Here's how the part is built. I have some questions about the finished solid (model axes, mm). Face numbers are marked on the shaded views. A direction names the side the tool comes from. Round coordinates to 2 decimals unless told otherwise and drop trailing zeros. Write each loop counter-clockwise with the first axis right and the second up, starting at its lowest first coordinate (ties: lowest second). Pieces come first, ordered by that corner, then holes. Notation, with made-up numbers: (55, 77) - (110, 77) arc R14 cw to (110, 91) - close; hole circle Ø10 at (-33, 88). An arc over 180 degrees is marked (long way). One line per item, written item: value. Start each with the question number.
Item 1: For P1, Ø7, axis at x = 0, z = 0, coming from the -Y side; P2, Ø2, axis at y = -2, z = 3, coming from the +X side; P3, Ø1, axis at x = 5, z = 7.5, coming from the +Y side, each with a flat end and sliding along its axis, tell me the tip position at first contact or that it passes through.
Item 2: Imagine slicing it at C-C, the plane y = 2.75. Please give me the cut outline in (x, z), then the cut area to 3 significant figures.
Item 3: If I drill on line 1 (X direction, y = -3.75, z = 0); line 2 (X direction, y = 2.5, z = 0); line 3 (Z direction, x = -7, y = 3.5), over which ranges is the centre line in solid material (lowest first)?
Item 4: Thinking about a two-plate mould opening in Z: for the marked faces 1, 2 and 3, which applies, released by +Z, released by -Z, zero draft, split by the parting line, or undercut?
Item 5: For the marked faces 4 and 5, which set-ups out of +Z, -Z, +X, -X, +Y, -Y let a thin tool reach every point of the face, with its end or its side?
Item 6: Imagine slicing it at D-D, the plane x = 4.75. Please give me the cut outline in (y, z).
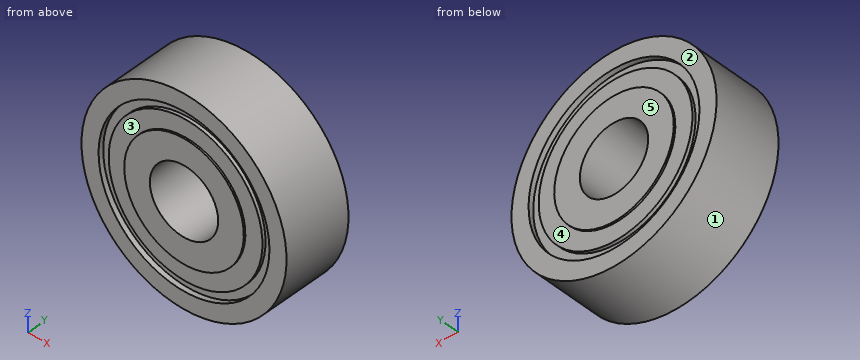
```python
from build123d import *

# Parameters (mm, degrees)
SKETCH1_R           = 7
SKETCH1_R_2         = 4
BOSS_EXTRUDE1_DEPTH = 4
SKETCH3_R           = 9
SKETCH3_R_2         = 7
BOSS_EXTRUDE2_DEPTH = 3.8
SKETCH4_R           = 10
SKETCH4_R_2         = 9
BOSS_EXTRUDE3_DEPTH = 3.4
SKETCH5_R           = 12
SKETCH5_R_2         = 10
BOSS_EXTRUDE4_DEPTH = 4


with BuildPart() as part:
    # Sketch1 → Boss-Extrude1 (new, symmetric)
    with BuildSketch(Plane(origin=(0, 0, 0), x_dir=(1, 0, 0), z_dir=(0, 1, 0))):
        with Locations(Location((0, 0, 0), (0, 0, 270))):
            Circle(SKETCH1_R)
        with Locations(Location((0, 0, 0), (0, 0, 270))):
            Circle(SKETCH1_R_2, mode=Mode.SUBTRACT)
    extrude(amount=BOSS_EXTRUDE1_DEPTH, both=True)

    # Sketch3 → Boss-Extrude2 (add, symmetric)
    with BuildSketch(Plane(origin=(0, 0, 0), x_dir=(1, 0, 0), z_dir=(0, 1, 0))):
        with Locations(Location((0, 0, 0), (0, 0, 90))):
            Circle(SKETCH3_R)
        with Locations(Location((0, 0, 0), (0, 0, 270))):
            Circle(SKETCH3_R_2, mode=Mode.SUBTRACT)
    extrude(amount=BOSS_EXTRUDE2_DEPTH, both=True)

    # Sketch4 → Boss-Extrude3 (add, symmetric)
    with BuildSketch(Plane(origin=(0, 0, 0), x_dir=(1, 0, 0), z_dir=(0, 1, 0))):
        with Locations(Location((0, 0, 0), (0, 0, 270))):
            Circle(SKETCH4_R)
        with Locations(Location((0, 0, 0), (0, 0, 90))):
            Circle(SKETCH4_R_2, mode=Mode.SUBTRACT)
    extrude(amount=BOSS_EXTRUDE3_DEPTH, both=True)

    # Sketch5 → Boss-Extrude4 (add, symmetric)
    with BuildSketch(Plane(origin=(0, 0, 0), x_dir=(1, 0, 0), z_dir=(0, 1, 0))):
        with Locations(Location((0, 0, 0), (0, 0, 270))):
            Circle(SKETCH5_R)
        with Locations(Location((0, 0, 0), (0, 0, 270))):
            Circle(SKETCH5_R_2, mode=Mode.SUBTRACT)
    extrude(amount=BOSS_EXTRUDE4_DEPTH, both=True)


solid = part.part
```
Values follow:
1. P1: passes through
1. P2: stops at x = 11.83
1. P3: stops at y = 3.8
2. outline: circle Ø24 at (0, 0); hole circle Ø8 at (0, 0)
2. area: 402 mm^2
3. line 1: x = -12 to -10, -9 to -4, 4 to 9, 10 to 12
3. line 2: x = -12 to -4, 4 to 12
3. line 3: z = -9.75 to -7.14, -5.66 to 5.66, 7.14 to 9.75
4. face 1: split by the parting line
4. face 2: zero draft
4. face 3: undercut
5. face 4: +Y
5. face 5: +Z, -Z, +X, -X, +Y
6. outline: (-4, -11.02) - (4, -11.02) - (4, -8.8) - (3.4, -8.8) - (3.4, -7.64) - (3.8, -7.64) - (3.8, -5.14) - (4, -5.14) - (4, 5.14) - (3.8, 5.14) - (3.8, 7.64) - (3.4, 7.64) - (3.4, 8.8) - (4, 8.8) - (4, 11.02) - (-4, 11.02) - (-4, 8.8) - (-3.4, 8.8) - (-3.4, 7.64) - (-3.8, 7.64) - (-3.8, 5.14) - (-4, 5.14) - (-4, -5.14) - (-3.8, -5.14) - (-3.8, -7.64) - (-3.4, -7.64) - (-3.4, -8.8) - (-4, -8.8) - close
